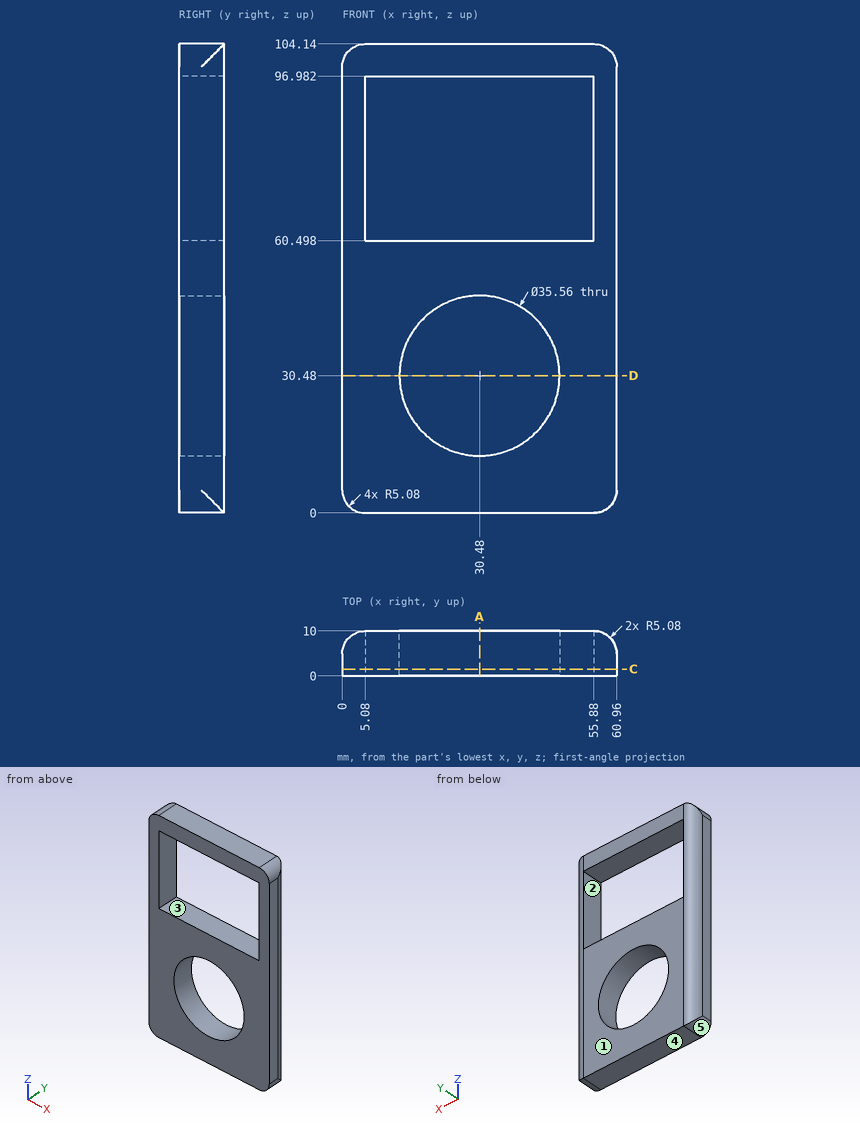
Here's the drawing with two shaded views (mm, measured from the low corner). I have some questions. A direction names the side the tool comes from. Coordinates: 2 decimals unless noted, no trailing zeros. Loops run counter-clockwise (first coordinate to the right, second up) from the corner with the lowest first, then second, coordinate; pieces in that order, holes last. Notation, with made-up numbers: M 56,31 L 100,31 A12 cw 100,48 Z; hole C 44.25,34 d1. An arc over 180 degrees is marked long. Answer as CSV lines item,"result". Start each with the question number.
1. Suppose I cut it at D-D, the plane z = 30.48. List the corners of the cut face in (x, y) for me.
2. If I drill on probe 1 along Z at (x, y) = (30.48, 7.25); probe 2 along X at (y, z) = (1.25, 70.5); probe 3 along Z at (x, y) = (39, 5) (1 decimal), over which ranges is the centre line in solid material (lowest first)? Write a range as [from, to].
3. Suppose I cut it at A-A, the plane x = 30.48. List the corners of the cut face in (y, z) for me.
4. Suppose I cut it at C-C, the plane y = 1.5. List the corners of the cut face in (x, z) for me.
5. For the marked faces 1 and 2, which set-ups out of +Z, -Z, +X, -X, +Y, -Y let a thin tool reach every point of the face, with its end or its side?
6. For pin 1 Ø1 at (y, z) = (5.5, 51.5) entering from +X, with a flat end and sliding along its axis, tell me the tip position at first contact or that it passes through.
7. Thinking about a two-plate mould opening in X: for the marked faces 3, 4 and 5, which applies, +X half, -X half, draft (parallel to the pull), parting line (faces both ways), or undercut?
Output:
1,outline,"M 0,0 L 12.7,0 L 12.7,10 L 5.08,10 A5.08 ccw 0,4.92 Z; M 48.26,0 L 60.96,0 L 60.96,4.92 A5.08 ccw 55.88,10 L 48.26,10 Z"
2,probe 1,"z = [0, 12.7], [48.26, 60.5], [96.98, 104.14]"
2,probe 2,"x = [0, 5.08], [55.88, 60.96]"
2,probe 3,"z = [0, 14.9], [46.1, 60.5], [97, 104.1]"
3,outline,"M 0,0 L 10,0 L 10,12.7 L 0,12.7 Z; M 0,48.26 L 10,48.26 L 10,60.5 L 0,60.5 Z; M 0,96.98 L 10,96.98 L 10,104.14 L 0,104.14 Z"
4,outline,"M 0,5.08 A5.08 ccw 5.08,0 L 55.88,0 A5.08 ccw 60.96,5.08 L 60.96,99.06 A5.08 ccw 55.88,104.14 L 5.08,104.14 A5.08 ccw 0,99.06 Z; hole M 5.08,60.5 L 55.88,60.5 L 55.88,96.98 L 5.08,96.98 Z; hole C 30.48,30.48 d35.56"
5,face 1,"+Z, -Z, +X, -X, +Y"
5,face 2,"+Y, -Y"
6,pin 1,"stops at x = 60.96"
7,face 3,"undercut"
7,face 4,"draft"
7,face 5,"-X half"
